from build123d import *

# Parameters (mm, degrees)
SKETCH2_W           = 300
SKETCH2_H           = 150
BOSS_EXTRUDE1_DEPTH = 60
SKETCH3_R           = 20


with BuildPart() as part:
    # Sketch2 → Boss-Extrude1 (new body)
    with BuildSketch(Plane(origin=(0, 0, 0), x_dir=(1, 0, 0), z_dir=(0, 1, 0))):
        Rectangle(SKETCH2_W, SKETCH2_H)
    extrude(amount=BOSS_EXTRUDE1_DEPTH)

    # Cut-Sweep3: sweep along a path in Sketch4
    with BuildLine(Plane(origin=(0, 60, 0), x_dir=(1, 0, 0), z_dir=(0, 1, 0))) as cut_sweep3_path:
        Line((-150, 75), (-150, -75))
        Line((-150, -75), (150, -75))
        Line((150, -75), (150, 75))
        Line((150, 75), (-150, 75))
    # Sketch3 → Cut-Sweep3 (sweep, cut)
    with BuildSketch(Plane.XY):
        with Locations((150, 60)):
            Circle(SKETCH3_R)
    sweep(path=cut_sweep3_path.line, transition=Transition.RIGHT, mode=Mode.SUBTRACT)


solid = part.part
Can you work these out from the model? Positions are in its coordinate system, mm. Give positions to 0.01 mm unless a question says otherwise; leave off trailing zeros. Loops run counter-clockwise (first coordinate to the right, second up) from the corner with the lowest first, then second, coordinate; pieces in that order, holes last. Notation, with made-up numbers: (57.25, -39.75) - (70.25, -39.75) arc R33 ccw to (70.25, -8.75) - close; hole circle Ø11 at (63.5, -21). An arc over 180 degrees is marked (long way). One line per item, written item: value.
(1) If we section it at C-C, the plane y = 55: List the corners of the cut face in (x, z) for me, plus the area to 3 significant figures.
Verdict:
outline: (-130.64, -55.64) - (130.64, -55.64) - (130.64, 55.64) - (-130.64, 55.64) - close
area: 29,100 mm^2
(2) I need wall thicknesses on line 1 along Z through (x, y) = (-78.5, 52); line 2 along X through (y, z) = (51, 7.5); line 3 along Z through (x, y) = (13.5, 45). Which ranges of each line are inside material? Lowest first, please.
Verdict:
line 1: -56.67 to 56.67
line 2: -132.14 to 132.14
line 3: -61.77 to 61.77
(3) I'm going to push flat-ended pins straight in: pin 1 (4 mm diameter, centred on y = 45, z = -22.5, fed in from -X); pin 2 (1.5 mm diameter, centred on x = 95.5, y = 53.5, fed in from +Z); pin 3 (4 mm diameter, centred on y = 51, z = 11, fed in from -X). Where does each tip first touch, or does it pass through?
Verdict:
pin 1: x = -139.46
pin 2: z = 56.36
pin 3: x = -133.3
(4) If we section it at B-B, the plane x = 73.5: List the corners of the cut face in (y, z) for me, plus the area to 3 significant figures.
Verdict:
outline: (0, -75) - (40, -75) arc R20 cw to (60, -55) - (60, 55) arc R20 cw to (40, 75) - (0, 75) - close
area: 8,370 mm^2
(5) If we section it at A-A, the plane z = -22: List the corners of the cut face in (x, y) for me.
Verdict:
outline: (-150, 0) - (150, 0) - (150, 40) arc R20 cw to (130, 60) - (-130, 60) arc R20 cw to (-150, 40) - close
